Verification items for the finished model (mm, model axes). Round coordinates to 2 decimals unless told otherwise and drop trailing zeros. Loops run counter-clockwise (first coordinate to the right, second up) from the corner with the lowest first, then second, coordinate; pieces in that order, holes last. Notation, with made-up numbers: (55.25, 33.5) -> (93.25, 33.5) arc R31 ccw to (93.25, 67.5) -> close; hole circle Ø2 at (50.5, -40). An arc over 180 degrees is marked (long way). Write item = value, one per line.
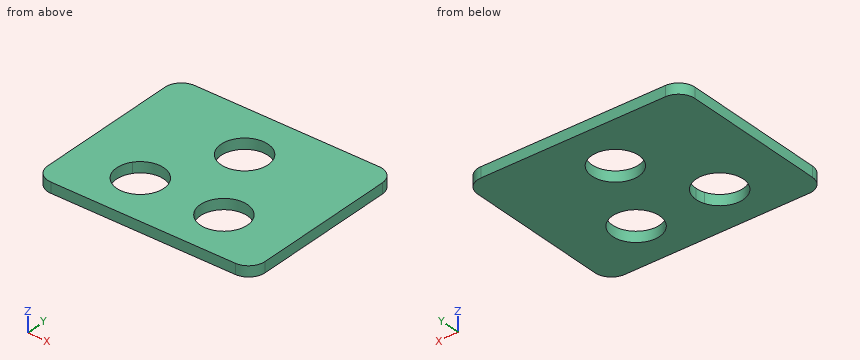
```python
from build123d import *
from build123d.topology import SkipClean

# Parameters (mm, degrees)
SKETCH1_R           = 14.2875
SKETCH1_R_2         = 53.34
BOSS_EXTRUDE1_DEPTH = 6.35


with BuildPart() as part:
    # Sketch1 → Boss-Extrude1 (new body)
    # profile 1 of 2: a face of its own
    with SkipClean():  # the faces are left unmerged after this step: merging them gives an invalid solid
        with BuildSketch(Plane.XY):
            with BuildLine():
                Line((-80.017343047, -25.364503898), (32.062656953, -25.364503898))
                ThreePointArc((32.062656953, -25.364503898), (39.133724765, -28.293436086), (42.062656953, -35.364503898))
                Line((42.062656953, -35.364503898), (42.062656953, -123.314503898))
                ThreePointArc((42.062656953, -123.314503898), (39.133724765, -130.38557171), (32.062656953, -133.314503898))
                Line((32.062656953, -133.314503898), (-80.017343047, -133.314503898))
                ThreePointArc((-80.017343047, -133.314503898), (-87.088410859, -130.38557171), (-90.017343047, -123.314503898))
                Line((-90.017343047, -123.314503898), (-90.017343047, -35.364503898))
                ThreePointArc((-90.017343047, -35.364503898), (-87.088410859, -28.293436086), (-80.017343047, -25.364503898))
            make_face()
            with Locations((-49.377343047, -104.018614592)):
                Circle(SKETCH1_R, mode=Mode.SUBTRACT)
            with Locations((-23.977343047, -57.114503898)):
                Circle(SKETCH1_R_2, mode=Mode.SUBTRACT)
            with Locations((1.422656953, -104.018614592)):
                Circle(SKETCH1_R, mode=Mode.SUBTRACT)
        # profile 2 of 2: a face of its own
        with BuildSketch(Plane.XY):
            with BuildLine():
                Line((18.883981011, -25.364503898), (-66.838667105, -25.364503898))
                ThreePointArc((-66.838667105, -25.364503898), (-77.128704465, -61.596510075), (-60.916565887, -95.593711477))
                ThreePointArc((-60.916565887, -95.593711477), (-44.94642836, -90.435549721), (-35.089843047, -104.018614592))
                ThreePointArc((-35.089843047, -104.018614592), (-35.3232221, -106.59045064), (-36.015735002, -109.078267418))
                ThreePointArc((-36.015735002, -109.078267418), (-23.977343047, -110.454503898), (-11.938951091, -109.078267418))
                ThreePointArc((-11.938951091, -109.078267418), (-5.380914475, -91.455013513), (12.961879794, -95.593711477))
                ThreePointArc((12.961879794, -95.593711477), (25.091454301, -78.028822602), (29.362656953, -57.114503898))
                ThreePointArc((29.362656953, -57.114503898), (26.67529077, -40.397258689), (18.883981011, -25.364503898))
            make_face()
            with Locations((-23.977343047, -57.114503898)):
                Circle(SKETCH1_R, mode=Mode.SUBTRACT)
        extrude(amount=BOSS_EXTRUDE1_DEPTH)


solid = part.part
```
(1) Sectioned sample at A-A, the plane x = -59.5. Record the cut outline in (y, z), and give its area (3 significant figures).
Filled sheet:
outline = (-133.31, 0) -> (-114.1, 0) -> (-114.1, 6.35) -> (-133.31, 6.35) -> close; (-93.94, 0) -> (-25.36, 0) -> (-25.36, 6.35) -> (-93.94, 6.35) -> close
area = 557 mm2
(2) Material ranges on probe 1 along X at (y, z) = (-48, 0.75); probe 2 along X at (y, z) = (-102, 2.5); probe 3 along Y at (x, z) = (-59, 4.5), recorded low to high. Write a range as from..to.
Filled sheet:
probe_1 = -90.02..-34.98, -12.97..42.06
probe_2 = -90.02..-63.52, -35.23..-12.72, 15.57..42.06
probe_3 = -133.31..-114.58, -93.46..-25.36
(3) Sectioned sample at B-B, the plane y = -63. Record the cut outline in (x, z), and give its area (3 significant figures).
Filled sheet:
outline = (-90.02, 0) -> (-37, 0) -> (-37, 6.35) -> (-90.02, 6.35) -> close; (-10.96, 0) -> (42.06, 0) -> (42.06, 6.35) -> (-10.96, 6.35) -> close
area = 673 mm2
(4) Sectioned sample at C-C, the plane z = 4.5. Record the cut outline in (x, y) (1 decimal).
Filled sheet:
outline = (-90, -123.3) arc R10 ccw to (-80, -133.3) -> (32.1, -133.3) arc R10 ccw to (42.1, -123.3) -> (42.1, -35.4) arc R10 ccw to (32.1, -25.4) -> (-80, -25.4) arc R10 ccw to (-90, -35.4) -> close; hole circle Ø28.6 at (-49.4, -104); hole circle Ø28.6 at (-24, -57.1); hole circle Ø28.6 at (1.4, -104)
